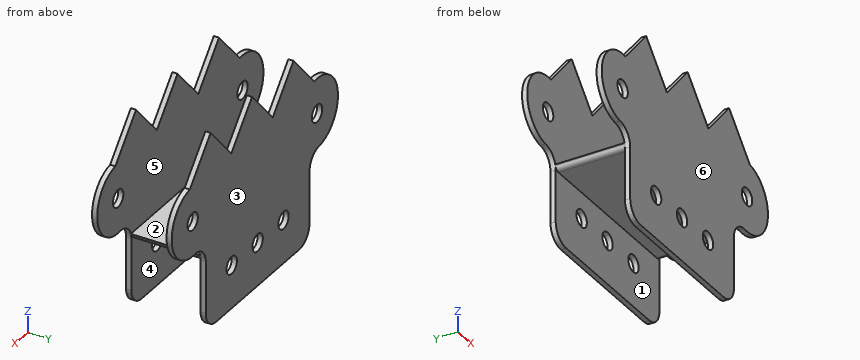
```python
from build123d import *

# Parameters (mm, degrees)
F0_R     = 5
F1_DEPTH = 46
F2_W     = 40
F2_H     = 62.4393149427
F2_H_2   = 108.6921231934
F3_DEPTH = 132.8823650188
F4_DEPTH = 27.4824745393
F5_R     = 3


with BuildPart() as f1:
    # F0 (on Front) → F1 (new body)
    with BuildSketch(Plane.XZ):
        with BuildLine():
            Line((-34.6001095204, 38.0689354645), (-54.6001095204, 15.7082556895))
            ThreePointArc((-54.6001095204, 15.7082556895), (-77.3000547602, -1.5917990707), (-60, -24.2917443105))
            ThreePointArc((-60, -24.2917443105), (-52.9289321881, -27.2206764986), (-50, -34.2917443105))
            Line((-50, -34.2917443105), (-50, -64.2917443105))
            ThreePointArc((-50, -64.2917443105), (-47.0710678119, -71.3628121224), (-40, -74.2917443105))
            Line((-40, -74.2917443105), (40, -74.2917443105))
            ThreePointArc((40, -74.2917443105), (47.0710678119, -71.3628121224), (50, -64.2917443105))
            Line((50, -64.2917443105), (50, -34.2917443105))
            ThreePointArc((50, -34.2917443105), (52.9289321881, -27.2206764986), (60, -24.2917443105))
            ThreePointArc((60, -24.2917443105), (82.6999452398, -6.9916895503), (65.3998904796, 15.7082556895))
            Line((65.3998904796, 15.7082556895), (45.3998904796, 38.0689354645))
            Line((45.3998904796, 38.0689354645), (25.3998904796, 15.7082556895))
            Line((25.3998904796, 15.7082556895), (5.3998904796, 38.0689354645))
            Line((5.3998904796, 38.0689354645), (-14.6001095204, 15.7082556895))
            Line((-14.6001095204, 15.7082556895), (-34.6001095204, 38.0689354645))
        make_face()
        with Locations((-25, -49.2917443105)):
            Circle(F0_R, mode=Mode.SUBTRACT)
        with Locations((0, -49.2917443105)):
            Circle(F0_R, mode=Mode.SUBTRACT)
        with Locations((25, -49.2917443105)):
            Circle(F0_R, mode=Mode.SUBTRACT)
        with Locations((-57.3000547602, -4.2917443105)):
            Circle(F0_R, mode=Mode.SUBTRACT)
        with Locations((62.6999452398, -4.2917443105)):
            Circle(F0_R, mode=Mode.SUBTRACT)
    extrude(amount=F1_DEPTH)

    # F2 (on face) → F3 (cut, through all)
    with BuildSketch(Plane(origin=(-50, 0, 0), x_dir=(0, -1, 0), z_dir=(-1, 0, 0))):
        with Locations((23, -65.5114017819)):
            Rectangle(F2_W, F2_H)
        with Locations((23, 23.0543172862)):
            Rectangle(F2_W, F2_H_2)
    extrude(amount=-F3_DEPTH, mode=Mode.SUBTRACT)

    # F2 (on face) → F4 (cut, through all)
    with BuildSketch(Plane(origin=(-50, 0, 0), x_dir=(0, -1, 0), z_dir=(-1, 0, 0))):
        with Locations((23, -65.5114017819)):
            Rectangle(F2_W, F2_H)
        with Locations((23, 23.0543172862)):
            Rectangle(F2_W, F2_H_2)
    extrude(amount=F4_DEPTH, mode=Mode.SUBTRACT)

    # F5
    f5_edges = [f1.edges().sort_by_distance(p)[0] for p in [
        (-50, -1.5, -34.291744),
        (-50, -23, -34.291744),
        (-50, -44.5, -34.291744),
        (50, -1.5, -34.291744),
        (50, -44.5, -34.291744),
        (50, -23, -34.291744),
    ]]
    fillet(f5_edges, radius=F5_R)


solid = f1.part
```
Check sheet for the modelled part. Datum: model origin and axes. Units: mm. Face numbers are marked on the shaded views. A direction names the side the tool comes from. Give positions to 0.01 mm unless a question says otherwise; leave off trailing zeros. Write each loop counter-clockwise with the first axis right and the second up, starting at its lowest first coordinate (ties: lowest second). Pieces come first, ordered by that corner, then holes. Notation, with made-up numbers: (88.5, 72) -> (132.5, 72) arc R25 ccw to (132.5, 85) -> close; hole circle Ø4 at (-1.75, 15.25). An arc over 180 degrees is marked (long way). Use CSV: the item, a comma, the result in double quotes. Start each with the question number.
Q1. Cross-section at B-B on x = 0. Enter the section's corners in (y, z).
Q2. Release check for a two-part mould opening along Y. For the marked faces 3, 4, 5 and 6 record: +Y half, -Y half, draft (parallel to the pull), parting line (faces both ways), or undercut.
Q3. Cross-section at D-D on y = -38.5. Enter the section's corners in (x, z).
Q4. Scan lines: line 1 along Y through (x, z) = (-62, -22.5); line 2 along Z through (x, y) = (-12, -37); line 3 along Z through (x, y) = (0, -1). Record each from-to range of solid material in increasing order.
Q5. Cross-section at C-C on z = 25.5. Enter the section's corners in (x, y).
Q6. Cross-section at A-A on z = -20. Enter the section's corners in (x, y).
Q7. Tool access check on the marked faces 1 and 2. Record the directions out of +Z, -Z, +X, -X, +Y, -Y that give a thin tool (end or side, any length) a straight path to the whole face; none if there is none.
Q8. Depth check by flat-ended pin: P1, Ø1.5, axis at y = -44, z = -55, coming from the +X side; P2, Ø12, axis at x = 8, z = -33.5, coming from the +Y side; P3, Ø12, axis at x = -19.5, y = -30.5, coming from the -Z side; P4, Ø1.5, axis at y = -2, z = -50.5, coming from the -X side. Enter the tip coordinate at first touch or a pass-through.
Working result:
1,outline,"(-46, -74.29) -> (-43, -74.29) -> (-43, -54.29) -> (-46, -54.29) -> close; (-46, -44.29) -> (-43, -44.29) -> (-43, -34.29) -> (-3, -34.29) -> (-3, -44.29) -> (0, -44.29) -> (0, 32.03) -> (-3, 32.03) -> (-3, -31.29) -> (-43, -31.29) -> (-43, 32.03) -> (-46, 32.03) -> close; (-3, -74.29) -> (0, -74.29) -> (0, -54.29) -> (-3, -54.29) -> close"
2,face 3,"+Y half"
2,face 4,"undercut"
2,face 5,"undercut"
2,face 6,"-Y half"
3,outline,"(-50.46, -31.29) arc R10 cw to (-50.27, -31.98) arc R3 ccw to (-47.35, -34.29) -> (47.35, -34.29) arc R3 ccw to (50.27, -31.98) arc R10 cw to (50.46, -31.29) -> close"
4,line 1,"y = -46 to -43, -3 to 0"
4,line 2,"z = -34.29 to -31.29"
4,line 3,"z = -74.29 to -54.29, -44.29 to 32.03"
5,outline,"(-45.84, -46) -> (-23.36, -46) -> (-23.36, -43) -> (-45.84, -43) -> close; (-45.84, -3) -> (-23.36, -3) -> (-23.36, 0) -> (-45.84, 0) -> close; (-5.84, -46) -> (16.64, -46) -> (16.64, -43) -> (-5.84, -43) -> close; (-5.84, -3) -> (16.64, -3) -> (16.64, 0) -> (-5.84, 0) -> close; (34.16, -46) -> (56.64, -46) -> (56.64, -43) -> (34.16, -43) -> close; (34.16, -3) -> (56.64, -3) -> (56.64, 0) -> (34.16, 0) -> close"
6,outline,"(-69.97, -46) -> (75.37, -46) -> (75.37, -43) -> (-69.97, -43) -> close; (-69.97, -3) -> (75.37, -3) -> (75.37, 0) -> (-69.97, 0) -> close"
7,face 1,"-Z, +X, -X"
7,face 2,"+Z, +X, -X"
8,P1,"stops at x = 50"
8,P2,"stops at y = 0"
8,P3,"stops at z = -34.29"
8,P4,"stops at x = -50"
